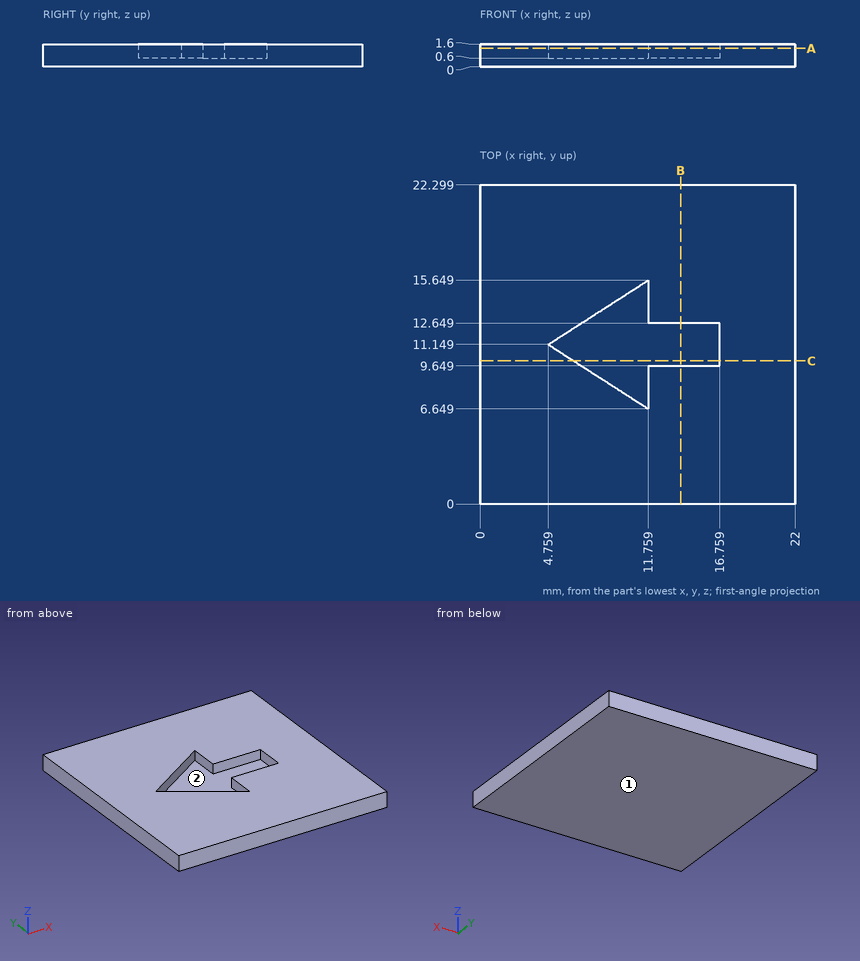
Design review of the part shown in the three views and the two pictorial views. Dimensions are in mm from the part's minimum x, y and z. Round coordinates to 2 decimals unless told otherwise and drop trailing zeros. Loops run counter-clockwise (first coordinate to the right, second up) from the corner with the lowest first, then second, coordinate; pieces in that order, holes last. Notation, with made-up numbers: (31, 66.5) -> (77, 66.5) arc R18 cw to (77, 78.5) -> close; hole circle Ø2 at (78, 69). An arc over 180 degrees is marked (long way). Use one line per item in the form item = value. Start each with the question number.
Q1. We need section A-A on z = 1.3. Give the boundary of the cut face in (x, y).
Q2. Draft analysis for pull direction X (two halves, no side actions). For the marked faces 1 and 2, state which applies: +X half, -X half, draft (parallel to the pull), parting line (faces both ways), or undercut.
Q3. We need section C-C on y = 10. Give the boundary of the cut face in (x, z).
Q4. For pin 1 Ø2.5 at (x, y) = (9.5, 10) entering from +Z, flat-tipped, find the tip position at first contact; note if it passes through.
Q5. We need section B-B on x = 14. Give the boundary of the cut face in (y, z).
Q6. Wall thickness on line 1 along Y through (x, z) = (16.25, 0.7); line 2 along Z through (x, y) = (9, 11.75); line 3 along X through (y, z) = (11, 1.15) (1 decimal): over which ranges is each line inside the solid? List them lowest first. Write a range as [from, to].
Calculated:
q1.outline = (0, 0) -> (22, 0) -> (22, 22.3) -> (0, 22.3) -> close; hole (4.76, 11.15) -> (11.76, 6.65) -> (11.76, 9.65) -> (16.76, 9.65) -> (16.76, 12.65) -> (11.76, 12.65) -> (11.76, 15.65) -> close
q2.face_1 = draft
q2.face_2 = undercut
q3.outline = (0, 0) -> (22, 0) -> (22, 1.6) -> (16.76, 1.6) -> (16.76, 0.6) -> (6.55, 0.6) -> (6.55, 1.6) -> (0, 1.6) -> close
q4.pin_1 = 0.6
q5.outline = (0, 0) -> (22.3, 0) -> (22.3, 1.6) -> (12.65, 1.6) -> (12.65, 0.6) -> (9.65, 0.6) -> (9.65, 1.6) -> (0, 1.6) -> close
q6.line_1 = [0, 9.65], [12.65, 22.3]
q6.line_2 = [0, 0.6]
q6.line_3 = [0, 5], [16.8, 22]
